Design review of the part built by this model. Coordinates are the model's own, in mm. Face numbers are marked on the shaded views. A direction names the side the tool comes from. Round coordinates to 2 decimals unless told otherwise and drop trailing zeros. Loops run counter-clockwise (first coordinate to the right, second up) from the corner with the lowest first, then second, coordinate; pieces in that order, holes last. Notation, with made-up numbers: (71.5, -2.75) -> (104.5, -2.75) arc R20 ccw to (104.5, 1.25) -> close; hole circle Ø3 at (25.25, 33). An arc over 180 degrees is marked (long way). Answer as CSV lines item,"result". Start each with the question number.
(1) Take a section at A-A, the plane y = 0. Write out the cut boundary in (x, z), and give its area (3 significant figures).
(2) Draft analysis for pull direction Z (two halves, no side actions). For the marked faces 1, 2 and 3, state which applies: +Z half, -Z half, draft (parallel to the pull), parting line (faces both ways), or undercut.
(3) Machinability: for the marked faces 4, 5 and 6, which of the approach directions +Z, -Z, +X, -X, +Y, -Y give a long, thin tool a straight path to every point of the face, cutting with its end or side? Answer none if there is none.
(4) Take a section at C-C, the plane x = 23. Write out the cut boundary in (y, z).
(5) Take a section at D-D, the plane x = 2.5. Write out the cut boundary in (y, z), and give its area (3 significant figures).
(6) To check wall thickness, follow line 1 (X direction, y = 6.25, z = 0); line 2 (Z direction, x = 11, y = 0); line 3 (Y direction, x = 21.5, z = 0). State the ranges of each line that lie inside material, in increasing order. Write a range as from..to.
(7) For P1, Ø1.5, axis at x = 22.5, z = 7, coming from the -Y side; P2, Ø6, axis at x = 27, y = 7.5, coming from the +Z side; P3, Ø1.5, axis at x = 9, y = 2, coming from the -Z side; P4, Ø4.5, axis at y = 0, z = 0, coming from the -X side, all flat-tipped, find the tip position at first contact; note any pin that passes through.
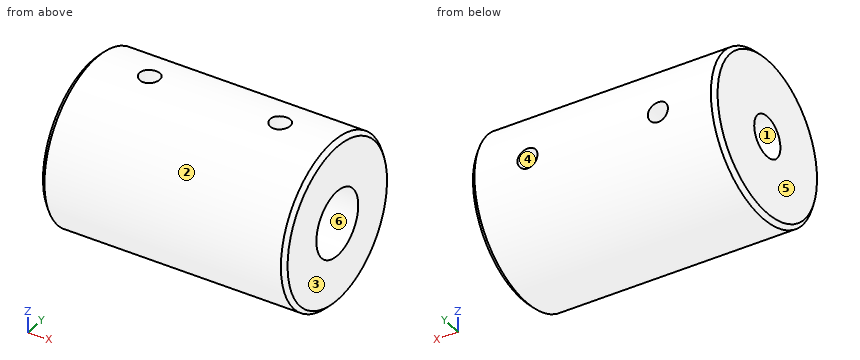
from build123d import *

# Parameters (mm, degrees)
SKETCH1_W          = 30
SKETCH1_H          = 10
SKETCH2_R          = 2.5
CUT_EXTRUDE1_DEPTH = 15
SKETCH3_R          = 4
CUT_EXTRUDE2_DEPTH = 15
TAP1_REACH         = 39.417
TAP1_BORE_R        = 1.2295
TAP2_REACH         = 39.417
TAP2_BORE_R        = 1.2295
CHAMFER1_SIZE      = 0.5


with BuildPart() as part:
    # Sketch1 → Revolve1 (revolve)
    with BuildSketch(Plane.XY, mode=Mode.PRIVATE) as revolve1_sk:
        with Locations((15, 5)):
            Rectangle(SKETCH1_W, SKETCH1_H)
    revolve(revolve1_sk.sketch.rotate(Axis((0, 0, 0), (1, 0, 0)), 90), axis=Axis((0, 0, 0), (1, 0, 0)))

    # Sketch2 → Cut-Extrude1 (cut)
    with BuildSketch(Plane(origin=(0, 0, 0), x_dir=(0, 0, -1), z_dir=(1, 0, 0))):
        Circle(SKETCH2_R)
    extrude(amount=CUT_EXTRUDE1_DEPTH, mode=Mode.SUBTRACT)

    # Sketch3 → Cut-Extrude2 (cut)
    with BuildSketch(Plane(origin=(30, 0, 0), x_dir=(0, 0, -1), z_dir=(1, 0, 0))):
        Circle(SKETCH3_R)
    extrude(amount=-CUT_EXTRUDE2_DEPTH, mode=Mode.SUBTRACT)

    # Tap1 bore → Tap1 (cut, up to next)
    with BuildSketch(Plane.XY.offset(10), mode=Mode.PRIVATE) as tap1_sk1:
        with Locations((7, 0)):
            Circle(TAP1_BORE_R)
    tap1_tool1 = extrude(tap1_sk1.sketch, amount=-TAP1_REACH, mode=Mode.PRIVATE) & part.part
    # Tap1 bore → Tap1 (cut, up to next)
    with BuildSketch(Plane.XY.offset(10), mode=Mode.PRIVATE) as tap1_sk2:
        with Locations((23, 0)):
            Circle(TAP1_BORE_R)
    tap1_tool2 = extrude(tap1_sk2.sketch, amount=-TAP1_REACH, mode=Mode.PRIVATE) & part.part
    add(tap1_tool1.solids().sort_by_distance((7, 0, 10))[0], mode=Mode.SUBTRACT)
    add(tap1_tool2.solids().sort_by_distance((23, 0, 10))[0], mode=Mode.SUBTRACT)

    # Tap2 bore → Tap2 (cut, up to next)
    with BuildSketch(Plane(origin=(0, 10, 0), x_dir=(1, 0, 0), z_dir=(0, 1, 0)), mode=Mode.PRIVATE) as tap2_sk1:
        with Locations((7, 0)):
            Circle(TAP2_BORE_R)
    tap2_tool1 = extrude(tap2_sk1.sketch, amount=-TAP2_REACH, mode=Mode.PRIVATE) & part.part
    # Tap2 bore → Tap2 (cut, up to next)
    with BuildSketch(Plane(origin=(0, 10, 0), x_dir=(1, 0, 0), z_dir=(0, 1, 0)), mode=Mode.PRIVATE) as tap2_sk2:
        with Locations((23, 0)):
            Circle(TAP2_BORE_R)
    tap2_tool2 = extrude(tap2_sk2.sketch, amount=-TAP2_REACH, mode=Mode.PRIVATE) & part.part
    add(tap2_tool1.solids().sort_by_distance((7, 10, 0))[0], mode=Mode.SUBTRACT)
    add(tap2_tool2.solids().sort_by_distance((23, 10, 0))[0], mode=Mode.SUBTRACT)

    # Chamfer1
    chamfer1_edges = [part.edges().sort_by_distance(p)[0] for p in [
        (30, 0, -10),
        (0, 0, -10),
    ]]
    chamfer(chamfer1_edges, length=CHAMFER1_SIZE)


solid = part.part
The answers:
1,outline,"(0, -9.5) -> (0.5, -10) -> (29.5, -10) -> (30, -9.5) -> (30, -4) -> (15, -4) -> (15, -2.5) -> (0, -2.5) -> close; (0, 2.5) -> (5.77, 2.5) -> (5.77, 10) -> (0.5, 10) -> (0, 9.5) -> close; (8.23, 2.5) -> (15, 2.5) -> (15, 4) -> (21.77, 4) -> (21.77, 10) -> (8.23, 10) -> close; (24.23, 4) -> (30, 4) -> (30, 9.5) -> (29.5, 10) -> (24.23, 10) -> close"
1,area,"371 mm²"
2,face 1,"undercut"
2,face 2,"parting line"
2,face 3,"draft"
3,face 4,"+Y"
3,face 5,"+Z, -Z, -X, +Y, -Y"
3,face 6,"+X"
4,outline,"(-1.23, 3.81) -> (-1.23, 9.92) arc R10 ccw (long way) to (9.92, -1.23) -> (3.81, -1.23) arc R4 cw (long way) to start; (1.23, 3.81) arc R4 cw to (3.81, 1.23) -> (9.92, 1.23) arc R10 ccw to (1.23, 9.92) -> close"
5,outline,"circle Ø20 at (0, 0); hole circle Ø5 at (0, 0)"
5,area,"295 mm²"
6,line 1,"0..5.77, 8.23..21.77, 24.23..30"
6,line 2,"-10..-2.5, 2.5..10"
6,line 3,"-10..-4, 4..10"
7,P1,"y = -7.81"
7,P2,"z = 8.93"
7,P3,"z = -9.92"
7,P4,"through"
